Geometry: final body of the model. Coordinates: model frame, mm. Round coordinates to 2 decimals unless told otherwise and drop trailing zeros. Loops run counter-clockwise (first coordinate to the right, second up) from the corner with the lowest first, then second, coordinate; pieces in that order, holes last. Notation, with made-up numbers: (54, -36) -> (92, -36) arc R8 cw to (92, -26) -> close; hole circle Ø1 at (-15.75, 59). An arc over 180 degrees is marked (long way). Answer in a Markdown table with one row per item.
```python
from build123d import *

# Parameters (mm, degrees)
F1_DEPTH = 10
F2_R     = 5
F3_R     = 3


with BuildPart() as f1:
    # F0 (on Top) → F1 (new body)
    with BuildSketch(Plane.XY):
        Polygon((-15.45085, 21.26627), (-25, -8.122992), (25, -8.122992), (15.45085, 21.26627), align=None)
    extrude(amount=F1_DEPTH)

    # F2
    f2_edges = [f1.edges().sort_by_distance(p)[0] for p in [
        (-15.45085, 21.26627, 5),
        (15.45085, 21.26627, 5),
    ]]
    fillet(f2_edges, radius=F2_R)

    # F3
    f3_edges = [f1.edges().sort_by_distance(p)[0] for p in [
        (-20.78671, 4.844181, 0),
        (-16.57342, 17.811355, 5),
        (-25, -8.122992, 5),
        (-20.78671, 4.844181, 10),
    ]]
    fillet(f3_edges, radius=F3_R)


solid = f1.part
```
Item 1: Section query A-A, the plane z = 3.5. Output: boundary loops of the cut face in (x, y).
Ans:
| item | result |
|---|---|
| outline | (-23.72, -4.2) arc R3 ccw to (-20.87, -8.12) -> (25, -8.12) -> (16.57, 17.81) arc R5 ccw to (11.82, 21.27) -> (-11.82, 21.27) arc R5 ccw to (-16.57, 17.81) -> close |
Item 2: Ray query, L1, parallel to Y at x = 9, z = 7.25; L2, parallel to X at y = -0.75, z = 9.5; L3, parallel to Z at x = 17, y = 12.75. Return the intervals inside material, ascending.
Ans:
| item | result |
|---|---|
| L1 | -8.12 to 21.26 |
| L2 | -21.19 to 21.19 |
| L3 | 0.63 to 9.37 |
Item 3: First-contact query: P1, Ø4, axis at y = 14.5, z = 1.5, coming from the +X side; P2, Ø4, axis at y = 2, z = 8, coming from the +X side; P3, Ø3, axis at y = -2, z = 7.5, coming from the -X side. Flat tips, straight axial feed; report the tip coordinate or a pass-through.
Ans:
| item | result |
|---|---|
| P1 | x = 18.17 |
| P2 | x = 22.3 |
| P3 | x = -23.48 |
